CAD build for the part. Positions are in the model's coordinates, mm. Face numbers are marked on the shaded views. A direction names the side the tool comes from. Round coordinates to 2 decimals unless told otherwise and drop trailing zeros. Order: outer loops, then holes, each group sorted by start corner. A loop starts at its lowest first (then second) coordinate and runs counter-clockwise, first axis right, second up. Notation, with made-up numbers: M -21.75,5.25 L 17.25,5.25 A17 cw 17.25,11.25 Z; hole C -34.5,-40 d10. An arc over 180 degrees is marked long. Answer as a JSON object with one key per item and string values.
```python
from build123d import *

# Parameters (mm, degrees)
F0_W           = 10
F0_H           = 10
F1_DEPTH       = 2.032
F2_DEPTH       = 4.064
F4_D           = 3.7973
F4_CSINK_D     = 7.7978
F4_CSINK_ANGLE = 82


with BuildPart() as f1:
    # F0 (on Front) → F1 (new body)
    with BuildSketch(Plane.XZ):
        with Locations((0, -3.175)):
            Rectangle(F0_W, F0_H)
    extrude(amount=F1_DEPTH)

    # F0 (on Front) → F2 (join)
    with BuildSketch(Plane.XZ):
        with Locations((0, 6.825)):
            Rectangle(F0_W, F0_H)
        with Locations((0, -3.175)):
            Rectangle(F0_W, F0_H)
    extrude(amount=-F2_DEPTH)

    # F4 (through all)
    with Locations(Plane(origin=(0, 4.064, 0), x_dir=(-1, 0, 0), z_dir=(0, 1, 0))):
        with Locations((0, -3.1738367397)):
            CounterSinkHole(F4_D / 2, F4_CSINK_D / 2, counter_sink_angle=F4_CSINK_ANGLE)


solid = f1.part
```
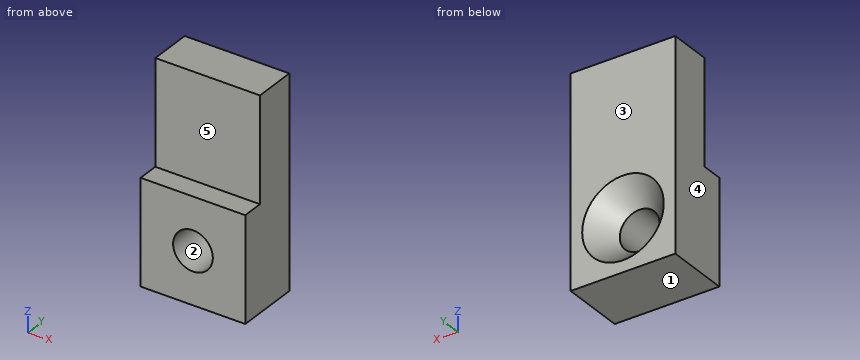
Item 1: Saw through at A-A on x = 0. List the corners of the cut face in (y, z) (3 decimals), and give its area (3 significant figures).
Worked answers:
{"outline": "M -2.032,-8.175 L 4.064,-8.175 L 4.064,-7.073 L 1.763,-5.072 L -2.032,-5.072 Z; M -2.032,-1.275 L 1.763,-1.275 L 4.064,0.725 L 4.064,11.825 L 0,11.825 L 0,1.825 L -2.032,1.825 Z", "area": "73.8 mm2"}
Item 2: Wall check: line 1 along Z through (x, y) = (0, -0.1) (3 decimals); line 2 along Z through (x, y) = (0, 0.6) (3 decimals); line 3 along Y through (x, z) = (-1, 9.5). Give the ranges that are in metal, low to high. Write a range as [from, to].
Worked answers:
{"line 1": "z = [-8.175, -5.072], [-1.275, 1.825]", "line 2": "z = [-8.175, -5.072], [-1.275, 11.825]", "line 3": "y = [0, 4.06]"}
Item 3: Saw through at B-B on y = 3.25. List the corners of the cut face in (x, z) (3 decimals), and give its area (3 significant figures).
Worked answers:
{"outline": "M -5,-8.175 L 5,-8.175 L 5,11.825 L -5,11.825 Z; hole C 0,-3.174 d6.383", "area": "168 mm2"}
Item 4: Saw through at C-C on z = 9.5. List the corners of the cut face in (x, y).
Worked answers:
{"outline": "M -5,0 L 5,0 L 5,4.06 L -5,4.06 Z"}
Item 5: Drop flat-ended pins along their axis: pin 1 Ø0.6 at (x, y) = (-1, -0.5) entering from +Z (3 decimals); pin 2 Ø3.5 at (x, z) = (0, -3.17) entering from +Y. Give the stop position or say it passes through.
Worked answers:
{"pin 1": "stops at z = 1.825", "pin 2": "passes through"}
Item 6: Two-plate mould, pull along Z, no slides. Class the marked faces 1, 2 and 3: released by +Z, released by -Z, zero draft, split by the parting line, or undercut.
Worked answers:
{"face 1": "released by -Z", "face 2": "undercut", "face 3": "zero draft"}
Item 7: 3-axis set-ups, long thin cutter, end or side, ignore diameter. For the marked faces 4 and 5: which of +Z, -Z, +X, -X, +Y, -Y reach the whole face in a straight line?
Worked answers:
{"face 4": "+Z, -Z, -X, +Y, -Y", "face 5": "+Z, +X, -X, -Y"}
Item 8: Saw through at D-D on y = 1.5. List the corners of the cut face in (x, z) (3 decimals).
Worked answers:
{"outline": "M -5,-8.175 L 5,-8.175 L 5,11.825 L -5,11.825 Z; hole C 0,-3.174 d3.797"}
